from build123d import *

# Parameters (mm, degrees)
F0_W      = 76.2
F0_H      = 63.5
F1_DEPTH  = 66.802
F2_W      = 63.5
F2_H      = 35.052
F2_H_2    = 19.05
F3_DEPTH  = 63.501
F4_R      = 12.7
F5_W      = 38.1
F5_H      = 6.35
F6_DEPTH  = 76.201
F8_DEPTH  = 12.701
F9_W      = 31.75
F9_H      = 7.874
F10_DEPTH = 31.751
F11_R     = 12.7
F12_DEPTH = 4.572
F13_R     = 7.112
F14_DEPTH = 27.179


with BuildPart() as f1:
    # F0 (on Top) → F1 (new body)
    with BuildSketch(Plane.XY):
        with Locations((38.1, 31.75)):
            Rectangle(F0_W, F0_H)
    extrude(amount=F1_DEPTH)

    # F2 (on face) → F3 (cut, through all)
    with BuildSketch(Plane.XZ):
        with Locations((44.45, 49.276)):
            Rectangle(F2_W, F2_H)
        with Locations((31.75, 9.525)):
            Rectangle(F2_W, F2_H_2)
    extrude(amount=-F3_DEPTH, mode=Mode.SUBTRACT)

    # F4
    f4_edges = [f1.edges().sort_by_distance(p)[0] for p in [
        (6.35, 0, 66.802),
        (6.35, 63.5, 66.802),
    ]]
    fillet(f4_edges, radius=F4_R)

    # F5 (on face) → F6 (cut, through all)
    with BuildSketch(Plane.YZ.offset(76.2)):
        with Locations((31.75, 3.175)):
            Rectangle(F5_W, F5_H)
    extrude(amount=-F6_DEPTH, mode=Mode.SUBTRACT)

    # F7 (on face) → F8 (cut, through all)
    with BuildSketch(Plane.YZ.offset(12.7)):
        with BuildLine():
            Line((50.799009, 61.976), (12.699009, 61.971204))
            ThreePointArc((12.699009, 61.971204), (4.830796, 54.102), (12.699009, 46.232796))
            Line((12.699009, 46.232796), (50.799009, 46.228))
            ThreePointArc((50.799009, 46.228), (58.674, 54.102), (50.799009, 61.976))
        make_face()
    extrude(amount=-F8_DEPTH, mode=Mode.SUBTRACT)

    # F9 (on face) → F10 (cut, through all)
    with BuildSketch(Plane.XY.offset(31.75)):
        with Locations((44.323, 59.563)):
            Rectangle(F9_W, F9_H)
        with Locations((44.323, 3.937)):
            Rectangle(F9_W, F9_H)
    extrude(amount=-F10_DEPTH, mode=Mode.SUBTRACT)

    # F11 (on face) → F12 (cut)
    with BuildSketch(Plane.XY.offset(31.75)):
        with Locations((44.323, 31.75)):
            Circle(F11_R)
    extrude(amount=-F12_DEPTH, mode=Mode.SUBTRACT)

    # F13 (on face) → F14 (cut, through all)
    with BuildSketch(Plane.XY.offset(27.178)):
        with Locations((44.323, 31.75)):
            Circle(F13_R)
    extrude(amount=-F14_DEPTH, mode=Mode.SUBTRACT)


solid = f1.part
Source: CAD feature listing. Evaluate the final solid. Frame: model axes, mm. A direction names the side the tool comes from. Give positions to 0.01 mm unless a question says otherwise; leave off trailing zeros. Write each loop counter-clockwise with the first axis right and the second up, starting at its lowest first coordinate (ties: lowest second). Pieces come first, ordered by that corner, then holes. Notation, with made-up numbers: M -31.5,11 L 10.5,11 A31 cw 10.5,47 Z; hole C 37.5,10 d8. An arc over 180 degrees is marked long. Answer as a JSON object with one key per item and string values.
Q1. Mould query, pull axis X, two halves, no side actions, for faces 4 (the face through (37.218, 32.063, 23.171)), 5 (the face through (76.2, 31, 16)), 6 (the face through (11, 63.5, 32)). Classes: +X half, -X half, draft (parallel to the pull), parting line (faces both ways), or undercut.
Geometry check:
{"face 4": "undercut", "face 5": "+X half", "face 6": "draft"}
Q2. Contact query for flat-ended pins moving along their axis: P1, Ø12, axis at x = 62.5, y = 35, coming from the +Z side; P2, Ø12, axis at x = 41.5, z = 29.5, coming from the -Y side; P3, Ø11.5, axis at x = 44.323, y = 31.75, coming from the -Z side; P4, Ø14, axis at x = 7, y = 26, coming from the -Z side. Output: stop coordinate, or through.
Geometry check:
{"P1": "stops at z = 31.75", "P2": "stops at y = 7.87", "P3": "passes through", "P4": "stops at z = 19.05"}
Q3. Access query for faces 1 (the face through (50, 26, 27.178)), 2 (the face through (28.448, 60, 25)), 3 (the face through (70, 12.7, 3)). Directions: +Z, -Z, +X, -X, +Y, -Y. A direction counts if a zero-diameter tool reaches every point of the face in a straight line with its end or side. Return the directions, or none.
Geometry check:
{"face 1": "+Z", "face 2": "+Z, -Z, +Y", "face 3": "-Z, +X, -X"}
Q4. Cut plane D-D, the plane z = 59. Return the cut outline in (x, y).
Geometry check:
{"outline": "M 0,0.98 L 12.7,0.98 L 12.7,6.54 L 0,6.54 Z; M 0,56.97 L 12.7,56.97 L 12.7,62.52 L 0,62.52 Z"}
Q5. Cut plane A-A, the plane z = 22.5. Return the cut outline in (x, y) (3 decimals).
Geometry check:
{"outline": "M 0,0 L 28.448,0 L 28.448,7.874 L 60.198,7.874 L 60.198,0 L 76.2,0 L 76.2,63.5 L 60.198,63.5 L 60.198,55.626 L 28.448,55.626 L 28.448,63.5 L 0,63.5 Z; hole C 44.323,31.75 d14.224"}
Q6. Cut plane B-B, the plane x = 6. Return the cut outline in (y, z).
Geometry check:
{"outline": "M 0,19.05 L 63.5,19.05 L 63.5,54.1 A12.7 ccw 50.8,66.8 L 12.7,66.8 A12.7 ccw 0,54.1 Z; hole M 12.7,46.23 L 50.8,46.23 A7.87 ccw 50.8,61.98 L 12.7,61.97 A7.87 ccw Z"}
Q7. Ray query, line 1 along Z through (x, y) = (10.5, 29); line 2 along Z through (x, y) = (18, 48); line 3 along X through (y, z) = (15, 42). Return the intervals inside material, ascending.
Geometry check:
{"line 1": "z = 19.05 to 46.23, 61.97 to 66.8", "line 2": "z = 19.05 to 31.75", "line 3": "x = 0 to 12.7"}
Q8. Cut plane C-C, the plane y = 29.5. Return the cut outline in (x, z), then the cut area to 3 significant figures.
Geometry check:
{"outline": "M 0,19.05 L 37.58,19.05 L 37.58,27.18 L 31.82,27.18 L 31.82,31.75 L 12.7,31.75 L 12.7,46.23 L 0,46.23 Z; M 0,61.97 L 12.7,61.97 L 12.7,66.8 L 0,66.8 Z; M 51.07,19.05 L 63.5,19.05 L 63.5,6.35 L 76.2,6.35 L 76.2,31.75 L 56.82,31.75 L 56.82,27.18 L 51.07,27.18 Z", "area": "1,150 mm^2"}
